```python
from build123d import *

# Parameters (mm, degrees)
SCHIZZO1_W                   = 56.4
SCHIZZO1_H                   = 9
SCHIZZO1_R                   = 1
ESTRUSIONE_ESTRUSIONE1_DEPTH = 3
SCHIZZO3_W                   = 14
SCHIZZO3_H                   = 13
ESTRUSIONE_ESTRUSIONE3_DEPTH = 2
FORO_PER_VITE_M2_1_D         = 2.4
FORO_PER_VITE_M2_1_DEPTH     = 56.4
TAGLIO_ESTRUSIONE1_DEPTH     = 1.56
SCHIZZO8_W                   = 9
SCHIZZO8_H                   = 1.5
TAGLIO_ESTRUSIONE2_DEPTH     = 1
SCHIZZO2_W                   = 52.4
SCHIZZO2_H                   = 2
ESTRUSIONE_ESTRUSIONE6_DEPTH = 1
SCHIZZO9_W                   = 9
SCHIZZO9_H                   = 2
TAGLIO_ESTRUSIONE3_DEPTH     = 2
TAGLIO_ESTRUSIONE5_START     = -29.09
SCHIZZO11_W                  = 13
SCHIZZO11_H                  = 0.6
TAGLIO_ESTRUSIONE5_DEPTH     = 74.965030919


with BuildPart() as part:
    # Schizzo1 → Estrusione-Estrusione1 (new body)
    with BuildSketch(Plane.XY):
        with Locations((0, -4.5)):
            Rectangle(SCHIZZO1_W, SCHIZZO1_H)
        with Locations((-23.725, -5.7)):
            Circle(SCHIZZO1_R, mode=Mode.SUBTRACT)
        with Locations(Location((23.725, -5.7, 0), (0, 0, 180))):
            Circle(SCHIZZO1_R, mode=Mode.SUBTRACT)
    extrude(amount=ESTRUSIONE_ESTRUSIONE1_DEPTH)

    # Schizzo3 → Estrusione-Estrusione3 (add)
    with BuildSketch(Plane(origin=(28.2, 0, 0), x_dir=(0, 0, -1), z_dir=(1, 0, 0))):
        with Locations((7, -6.5)):
            Rectangle(SCHIZZO3_W, SCHIZZO3_H)
    estrusione_estrusione3 = extrude(amount=-ESTRUSIONE_ESTRUSIONE3_DEPTH)

    # Foro per Vite M2-1
    with Locations(Plane(origin=(28.2, 0, 0), x_dir=(0, 0, -1), z_dir=(1, 0, 0))):
        with Locations((4.5, -9.64)):
            foro_per_vite_m2_1 = Hole(FORO_PER_VITE_M2_1_D / 2, depth=FORO_PER_VITE_M2_1_DEPTH)

    # Schizzo6 → Taglio-Estrusione1 (cut)
    with BuildSketch(Plane.ZY.offset(-26.2)):
        Polygon((-3.359733218, -7.665), (-5.640266782, -7.665), (-6.780533563, -9.64), (-5.640266782, -11.615), (-3.359733218, -11.615), (-2.219466437, -9.64), align=None)
    taglio_estrusione1 = extrude(amount=-TAGLIO_ESTRUSIONE1_DEPTH, mode=Mode.SUBTRACT)

    # Specchia2: Estrusione-Estrusione3, Foro per Vite M2-1, Taglio-Estrusione1 across plane
    add(estrusione_estrusione3.mirror(Plane(origin=(0, 0, 0), x_dir=(0, 0, 1), z_dir=(1, 0, 0))))
    add(foro_per_vite_m2_1.mirror(Plane(origin=(0, 0, 0), x_dir=(0, 0, 1), z_dir=(1, 0, 0))), mode=Mode.SUBTRACT)
    add(taglio_estrusione1.mirror(Plane(origin=(0, 0, 0), x_dir=(0, 0, 1), z_dir=(1, 0, 0))), mode=Mode.SUBTRACT)

    # Schizzo8 → Taglio-Estrusione2 (cut)
    with BuildSketch(Plane.XY):
        with Locations((9, -4.44)):
            Rectangle(SCHIZZO8_W, SCHIZZO8_H)
    extrude(amount=TAGLIO_ESTRUSIONE2_DEPTH, mode=Mode.SUBTRACT)

    # Schizzo2 → Estrusione-Estrusione6 (add)
    with BuildSketch(Plane(origin=(0, 0, 0), x_dir=(-1, 0, 0), z_dir=(0, 0, -1))):
        with Locations((0, -1)):
            Rectangle(SCHIZZO2_W, SCHIZZO2_H)
    extrude(amount=ESTRUSIONE_ESTRUSIONE6_DEPTH)

    # Schizzo9 → Taglio-Estrusione3 (cut)
    with BuildSketch(Plane(origin=(0, 0, 0), x_dir=(1, 0, 0), z_dir=(0, 1, 0))):
        Rectangle(SCHIZZO9_W, SCHIZZO9_H)
    extrude(amount=-TAGLIO_ESTRUSIONE3_DEPTH, mode=Mode.SUBTRACT)

    # Schizzo11 → Taglio-Estrusione5 (cut, through all)
    with BuildSketch(Plane(origin=(0, -32.78, -9), x_dir=(-1, 0, 0), z_dir=(0, -1, 0)).offset(TAGLIO_ESTRUSIONE5_START)):
        with Locations((15, -10.3)):
            Rectangle(SCHIZZO11_W, SCHIZZO11_H)
        with Locations((-15, -10.3)):
            Rectangle(SCHIZZO11_W, SCHIZZO11_H)
    extrude(amount=TAGLIO_ESTRUSIONE5_DEPTH, mode=Mode.SUBTRACT)


solid = part.part
```
Geometry check sheet. Reference: the model listing, model coordinates, mm. A direction names the side the tool comes from. Round coordinates to 2 decimals unless told otherwise and drop trailing zeros. Loops run counter-clockwise (first coordinate to the right, second up) from the corner with the lowest first, then second, coordinate; pieces in that order, holes last. Notation, with made-up numbers: (12, -21.75) -> (26, -21.75) arc R10 ccw to (26, -13.75) -> close; hole circle Ø8 at (-22.75, 47.5). An arc over 180 degrees is marked (long way). Use a Markdown table: item, result.
(1) Sectioned sample at D-D (z = -11.25). Enter the section's corners in (x, y), then the cut area to 3 significant figures.
Calculated:
| item | result |
|---|---|
| outline | (-28.2, -13) -> (-26.2, -13) -> (-26.2, 0) -> (-28.2, 0) -> close; (26.2, -13) -> (28.2, -13) -> (28.2, 0) -> (26.2, 0) -> close |
| area | 52.0 mm² |
(2) Mould release check, pull along X, two halves, no side actions. Record for faces 1 (the flat face through (27, -13, -7)), 2 (the flat face through (-28.2, -6, -5)), 3 (the flat face through (11, -3.69, 1)): released by +X, released by -X, zero draft, split by the parting line, or undercut.
Calculated:
| item | result |
|---|---|
| face 1 | zero draft |
| face 2 | released by -X |
| face 3 | undercut |
(3) Sectioned sample at A-A (y = -5.7). Enter the section's corners in (x, z) (3 decimals), then the cut area to 3 significant figures.
Calculated:
| item | result |
|---|---|
| outline | (-28.2, -14) -> (-26.2, -14) -> (-26.2, 0) -> (-24.725, 0) -> (-24.725, 3) -> (-28.2, 3) -> close; (-22.725, 0) -> (22.725, 0) -> (22.725, 3) -> (-22.725, 3) -> close; (24.725, 0) -> (26.2, 0) -> (26.2, -14) -> (28.2, -14) -> (28.2, 3) -> (24.725, 3) -> close; hole (-21.5, 1) -> (-8.5, 1) -> (-8.5, 1.6) -> (-21.5, 1.6) -> close; hole (8.5, 1) -> (21.5, 1) -> (21.5, 1.6) -> (8.5, 1.6) -> close |
| area | 198 mm² |
(4) Set-up check for faces 4 (the flat face through (-26.97, -10.61, -6.22)), 5 (the flat face through (-15, -6, 1.6)), 6 (the flat face through (-15, -1, -1)), 7 (the flat face through (8.9, -5.19, 0.5)): record each of +Z, -Z, +X, -X, +Y, -Y from which the full face is reachable in a straight line by a thin tool's end or side.
Calculated:
| item | result |
|---|---|
| face 4 | none |
| face 5 | -Y |
| face 6 | -Z, +Y, -Y |
| face 7 | -Z |
(5) Sectioned sample at C-C (x = 19.5). Enter the section's corners in (y, z).
Calculated:
| item | result |
|---|---|
| outline | (-9, 0) -> (-2, 0) -> (-2, -1) -> (0, -1) -> (0, 3) -> (-9, 3) -> (-9, 1.6) -> (-3.69, 1.6) -> (-3.69, 1) -> (-9, 1) -> close |
(6) Scan lines: probe 1 along X at (y, z) = (-12, -2.75); probe 2 along Y at (x, z) = (-28.05, -4.5); probe 3 along Z at (x, y) = (13, -7.25). Record each from-to range of solid material in increasing order.
Calculated:
| item | result |
|---|---|
| probe 1 | -28.2 to -26.2, 26.2 to 28.2 |
| probe 2 | -13 to -10.84, -8.44 to 0 |
| probe 3 | 0 to 1, 1.6 to 3 |
(7) Sectioned sample at B-B (z = -4.5). Enter the section's corners in (x, y) (3 decimals), then the cut area to 3 significant figures.
Calculated:
| item | result |
|---|---|
| outline | (-28.2, -13) -> (-26.2, -13) -> (-26.2, -11.615) -> (-27.76, -11.615) -> (-27.76, -10.84) -> (-28.2, -10.84) -> close; (-28.2, -8.44) -> (-27.76, -8.44) -> (-27.76, -7.665) -> (-26.2, -7.665) -> (-26.2, 0) -> (-28.2, 0) -> close; (26.2, -13) -> (28.2, -13) -> (28.2, -10.84) -> (27.76, -10.84) -> (27.76, -11.615) -> (26.2, -11.615) -> close; (26.2, -7.665) -> (27.76, -7.665) -> (27.76, -8.44) -> (28.2, -8.44) -> (28.2, 0) -> (26.2, 0) -> close |
| area | 37.6 mm² |
(8) Go/stop test with flat-tipped pins: P1, Ø1.9, axis at y = -9.64, z = -4.5, coming from the -X side; P2, Ø0.5, axis at x = -13.5, z = 1, coming from the -Y side; P3, Ø0.6, axis at x = -19.5, y = -1, coming from the -Z side; P4, Ø4, axis at x = 12, y = -6, coming from the -Z side. Record where each tip stops, or that it passes through.
Calculated:
| item | result |
|---|---|
| P1 | through |
| P2 | y = -9 |
| P3 | z = -1 |
| P4 | z = 0 |
